Autodesk Fusion 360 part; units mm, degrees
sketch "3D-printed conduit outline" plane through (0, 0, 0) normal (0, 1, 0) x (1, 0, 0)
  line L0 (0, 0) -> (16, 0)
  line L1 (16, 0) -> (16, -14)
  line L2 (16, -14) -> (0, -14)
  line L3 (0, -14) -> (0, 0)
  line L4 (2, -14) -> (14, -14)
  line L5 (14, -14) -> (14, -2)
  line L6 (14, -2) -> (2, -2)
  line L7 (2, -2) -> (2, -14)
  dimension "d8" = 14
  dimension "d9" = 16
  dimension "d10" = 2
  dimension "d11" = 2
  dimension "d12" = 2
extrude "Extrude1" add sketch "3D-printed conduit outline" along normal blind 69.355 contours L0 L1 L2 L3 L5 L6 L7
sketch "Magnet holders" plane through (0, 0, 14) normal (0, 0, 1) x (-1, 0, 0)
  line L0 (0, 0) -> (-2, 0)
  line L1 (-2, 0) -> (-2, -69.355)
  line L2 (-2, -69.355) -> (0, -69.355)
  line L3 (0, -69.355) -> (0, 0)
  line L4 (-14, 0) -> (-16, 0)
  line L5 (-16, 0) -> (-16, -69.355)
  line L6 (-16, -69.355) -> (-14, -69.355)
  line L7 (-14, -69.355) -> (-14, 0)
  circle A0 centre (-2.5, -2.5) radius 2.5
  circle A1 centre (-2.5, -2.5) radius 1.75
  line L8 (-14, 0) -> (-2, 0)
  line L9 (0, 0) -> (-2.5, 0)
  line L10 (-2.5, 0) -> (-2.5, -5)
  line L11 (-2.5, -5) -> (0, -5)
  line L12 (0, -5) -> (0, 0)
  circle A2 centre (-13.5, -2.5) radius 2.5
  circle A3 centre (-13.5, -2.5) radius 1.75
  line L13 (-16, 0) -> (-13.5, 0)
  line L14 (-13.5, 0) -> (-13.5, -5)
  line L15 (-13.5, -5) -> (-16, -5)
  line L16 (-16, -5) -> (-16, 0)
  circle A4 centre (-2.5, -50.855) radius 1.75
  circle A5 centre (-2.5, -50.855) radius 2.5
  line L17 (-2.5, -48.355) -> (-2.5, -53.355)
  line L18 (-2.5, -53.355) -> (0, -53.355)
  line L19 (0, -53.355) -> (0, -48.355)
  line L20 (0, -48.355) -> (-2.5, -48.355)
  circle A6 centre (-13.5, -66.855) radius 2.5
  circle A7 centre (-13.5, -66.855) radius 1.75
  line L21 (-13.5, -64.355) -> (-13.5, -69.355)
  line L22 (-13.5, -69.355) -> (-16, -69.355)
  line L23 (-16, -69.355) -> (-16, -64.355)
  line L24 (-16, -64.355) -> (-13.5, -64.355)
  dimension "d15" = 5
  dimension "d16" = 3.5
  dimension "d17" = 5
  dimension "d18" = 3.5
  dimension "d21" = 0
  dimension "d22" = -48.355
  dimension "d42" = 0
  dimension "d43" = -64.355
sketch "End wall" plane through (0, 69.355, 0) normal (0, 1, 0) x (-1, 0, 0)
  line L0 (-2, 2) -> (-14, 2)
  line L1 (-14, 2) -> (-14, 14)
  line L2 (-14, 14) -> (-16, 14)
  line L3 (-16, 14) -> (-16, 0)
  line L4 (-16, 0) -> (0, 0)
  line L5 (0, 0) -> (0, 14)
  line L6 (0, 14) -> (-2, 14)
  line L7 (-2, 14) -> (-2, 2)
  line L8 (-16, 0) -> (0, 0)
  line L9 (0, 0) -> (0, 14)
  line L10 (0, 14) -> (-16, 14)
  line L11 (-16, 14) -> (-16, 0)
extrude "Extrude8" add sketch "End wall" against normal blind 2
extrude "Extrude2" add sketch "Magnet holders" against normal blind 3 contours A2 A3 L14 | L7 A2 A3 L14 | L7 L8 A2 L13 | L1 A0 L8 L9 | L1 A0 A1 L10 | A0 A1 L10 | L1 A0 A1 L10 | L1 A0 L11 | L1 A1 L10 | A1 L10 | L7 A3 L14 | A3 L14 | L1 A5 L20 | L7 A2 L15 | L7 A2 A3 L14 | L1 A4 A5 L17 | L1 A4 A5 L17 | L1 A5 L18 | A4 A5 L17 | L1 A4 L17 | A4 L17 | L7 A6 L24 | L7 A6 A7 L21 | A6 A7 L21 | L7 A7 L21 | A7 L21 | L7 A6 L22 | L7 A6 A7 L21
extrude "Extrude4" cut sketch "Magnet holders" against normal blind 1 contours L1 A1 | L1 A1 L10 | A1 L10 | L7 A3 L14 | A3 L14 | L7 A3 | L1 A4 | L1 A4 L17 | A4 L17 | L7 A7 L21 | L7 A7 | A7 L21
chamfer "Chamfer2" distance 2.9999 angle 45 5 edges at (2, 2.5, 11) (2, 50.855, 11) (2, 2.5, 11) (14, 2.5, 11) (14, 65.855, 11)
sketch "Smartie hopper mechanism conduit 2 outlet" plane through (0, 0, 0) normal (-1, 0, 0) x (0, -1, 0)
  line L0 (-69.355, 0) -> (0, 0)
  line L1 (0, 0) -> (0, 14)
  line L2 (0, 14) -> (-69.355, 14)
  line L3 (-69.355, 14) -> (-69.355, 0)
  line L4 (-67.355, 14) -> (-55.355, 14)
  line L5 (-55.355, 14) -> (-55.355, 2)
  line L6 (-55.355, 2) -> (-67.355, 2)
  line L7 (-67.355, 2) -> (-67.355, 14)
  dimension "d60" = 2
  dimension "d61" = 12
  dimension "d62" = 2
extrude "Extrude11" cut sketch "Smartie hopper mechanism conduit 2 outlet" against normal blind 2 contours L2 L4 L5 L6 L7
chamfer "Chamfer5" distance 1 angle 45 4 edges at (2, 27.6775, 2) (1, 55.355, 2) (7, 67.355, 2) (14, 33.6775, 2)
equation "conduit_length = 69.355 mm"
equation "conduit_width = 16 mm"
equation "conduit_height = 16 mm"
equation "conduit_wall_thickness = 2 mm"
equation "magnet_diameter = 3 mm"
equation "magnet_height = 1 mm"
equation "d8 = conduit_height - conduit_wall_thickness"
equation "d9 = conduit_width"
equation "d10 = conduit_wall_thickness"
equation "d11 = conduit_wall_thickness"
equation "d12 = conduit_wall_thickness"
equation "d13 = conduit_length"
equation "d15 = magnet_diameter + 2 mm"
equation "d16 = magnet_diameter + 0.5 mm"
equation "d17 = magnet_diameter + 2 mm"
equation "d18 = magnet_diameter + 0.5 mm"
equation "d22 = -conduit_length + ( magnet_diameter + 2 mm ) + ( conduit_width )"
equation "d23 = -( magnet_height + 2 mm )"
equation "d43 = -conduit_length + ( magnet_diameter + 2 mm )"
equation "d60 = conduit_wall_thickness"
equation "d62 = conduit_wall_thickness"
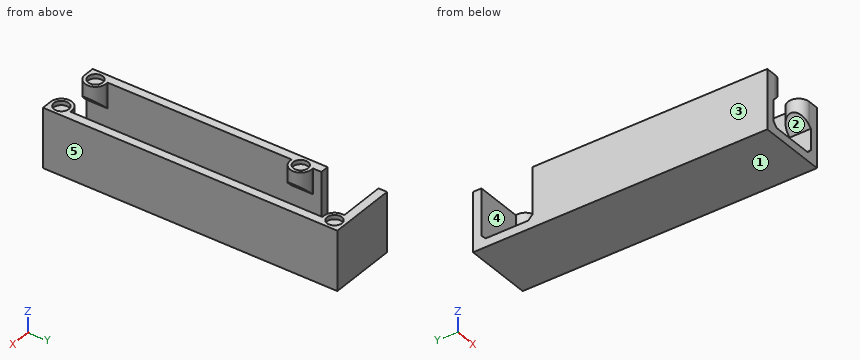
Read the model definition and answer for the solid it produces. Units are mm, in the model's axes. Face numbers are marked on the shaded views. A direction names the side the tool comes from. Give positions to 0.01 mm unless a question says otherwise; leave off trailing zeros. Write each loop counter-clockwise with the first axis right and the second up, starting at its lowest first coordinate (ties: lowest second). Pieces come first, ordered by that corner, then holes. Notation, with made-up numbers: (48, 28) -> (88, 28) arc R26 ccw to (88, 46) -> close; hole circle Ø6 at (16, -27). An arc over 180 degrees is marked (long way). Answer as a JSON object with one key per item and string values. Group by question number.
1) Find section A-A (z = 5). Write down the section's boundary in (x, y) (3 decimals), and give its area (3 significant figures).
2) Consider L1, parallel to Y at x = 13.5, z = 13.6 (3 decimals); L2, parallel to X at y = 2.5, z = 13.35; L3, parallel to X at y = 15, z = 10.5. Determine where each line is inside the solid, lowest interval first. Write a range as from..to.
3) A tool of negligible diameter and unlimited length cuts with its end or side. For the marked faces 4 and 5, from which of +Z, -Z, +X, -X, +Y, -Y can it reach the whole face along a straight path? Write none if from no direction.
4) Find section B-B (x = 7.75). Write down the section's boundary in (y, z) (3 decimals).
5) Find section C-C (y = 13.5). Write down the section's boundary in (x, z).
6) Find section D-D (z = 9.75). Write down the section's boundary in (x, y) (3 decimals), and give its area (3 significant figures).
7) The mould has two halves that part along Z. Classify the marked faces 1, 2 and 3: +Z half, -Z half, draft (parallel to the pull), parting line (faces both ways), or undercut.
8) Each of these flat-tipped pins is pushed along its axis until it touches: P1, Ø4, axis at x = 2.5, y = 2.5, coming from the +Z side; P2, Ø6, axis at x = 9, z = 6.5, coming from the -Y side (3 decimals); P3, Ø1, axis at x = 13.5, y = 2, coming from the +Z side. Where does it stop, or does it pass through?
Values follow:
{
 "1": {"outline": "(0, 0) -> (2, 0) -> (2, 55.355) -> (0, 55.355) -> close; (0, 67.355) -> (14, 67.355) -> (14, 0) -> (16, 0) -> (16, 69.355) -> (0, 69.355) -> close", "area": "277 mm2"},
 "2": {"L1": "y = 0..0.75, 4.25..5, 64.355..65.105, 68.605..69.355", "L2": "x = 0..0.75, 4.25..5, 11..11.75, 15.25..16", "L3": "x = 0..2, 14..16"},
 "3": {"face 4": "-X", "face 5": "+Z, -Z, +X, +Y, -Y"},
 "4": {"outline": "(0, 0) -> (69.355, 0) -> (69.355, 14) -> (67.355, 14) -> (67.355, 3) -> (66.355, 2) -> (0, 2) -> close"},
 "5": {"outline": "(0, 0) -> (16, 0) -> (16, 14) -> (14, 14) -> (14, 3) -> (13, 2) -> (3, 2) -> (2, 3) -> (2, 14) -> (0, 14) -> close"},
 "6": {"outline": "(0, 0) -> (2.5, 0) arc R2.5 ccw to (3.75, 0.335) -> (3.75, 4.665) arc R2.5 ccw to (2.5, 5) -> (2, 5) -> (2, 48.355) -> (2.5, 48.355) arc R2.5 ccw to (3.75, 48.69) -> (3.75, 53.02) arc R2.5 ccw to (2.5, 53.355) -> (2, 53.355) -> (2, 55.355) -> (0, 55.355) -> close; (0, 67.355) -> (12.25, 67.355) -> (12.25, 64.69) arc R2.5 ccw to (13.5, 64.355) -> (14, 64.355) -> (14, 5) -> (13.5, 5) arc R2.5 ccw to (12.25, 4.665) -> (12.25, 0.335) arc R2.5 ccw to (13.5, 0) -> (16, 0) -> (16, 69.355) -> (0, 69.355) -> close", "area": "308 mm2"},
 "7": {"face 1": "-Z half", "face 2": "undercut", "face 3": "draft"},
 "8": {"P1": "stops at z = 14", "P2": "stops at y = 67.355", "P3": "stops at z = 13"}
}
